from build123d import *

# Parameters (mm, degrees)
SKETCH003_R      = 2
EXTRUDE003_DEPTH = 1.5
SKETCH004_R      = 4
EXTRUDE004_DEPTH = 1.5
EXTRUDE001_DEPTH = 3
SKETCH002_W      = 30
SKETCH002_H      = 30
SKETCH002_R      = 7.071068
EXTRUDE002_DEPTH = 3
SKETCH_W         = 30
SKETCH_H         = 30
EXTRUDE_DEPTH    = 3


with BuildPart() as furo:
    # Sketch003 → Extrude003 (new body)
    with BuildSketch(Plane.XY):
        with Locations((15, 21)):
            Circle(SKETCH003_R)
        with Locations((15, 9)):
            Circle(SKETCH003_R)
    extrude(amount=EXTRUDE003_DEPTH)


with BuildPart() as fusion:
    # Sketch004 → Extrude004 (new body)
    with BuildSketch(Plane.XY.offset(1.5)):
        with Locations((15, 21)):
            Circle(SKETCH004_R)
        with Locations((15, 9)):
            Circle(SKETCH004_R)
    extrude(amount=EXTRUDE004_DEPTH)

    # Fusion: union Furo
    add(furo.part)


with BuildPart() as lateral:
    # Sketch001 → Extrude001 (new body)
    with BuildSketch(Plane.XZ):
        Polygon((0, 3), (0, 30), (30, 3), align=None)
    extrude(amount=-EXTRUDE001_DEPTH)


with BuildPart() as lateral_mirrored:
    # mirror: instance of Lateral
    add(lateral.part.mirror(Plane(origin=(30, 15, 0), x_dir=(-1, 0, 0), z_dir=(0, -1, 0))))


with BuildPart() as frontal:
    # Sketch002 → Extrude002 (new body)
    with BuildSketch(Plane.YZ):
        with Locations((15, 15)):
            Rectangle(SKETCH002_W, SKETCH002_H)
        with Locations((15, 15)):
            Circle(SKETCH002_R, mode=Mode.SUBTRACT)
    extrude(amount=-EXTRUDE002_DEPTH)


with BuildPart() as cut:
    # Sketch → Extrude (new body)
    with BuildSketch(Plane.XY):
        with Locations((15, 15)):
            Rectangle(SKETCH_W, SKETCH_H)
    extrude(amount=EXTRUDE_DEPTH)

    # Fusion001: union Lateral (mirrored), Lateral, Frontal
    add(lateral_mirrored.part)
    add(lateral.part)
    add(frontal.part)

    # Cut: cut Fusion
    add(fusion.part, mode=Mode.SUBTRACT)


solid = cut.part
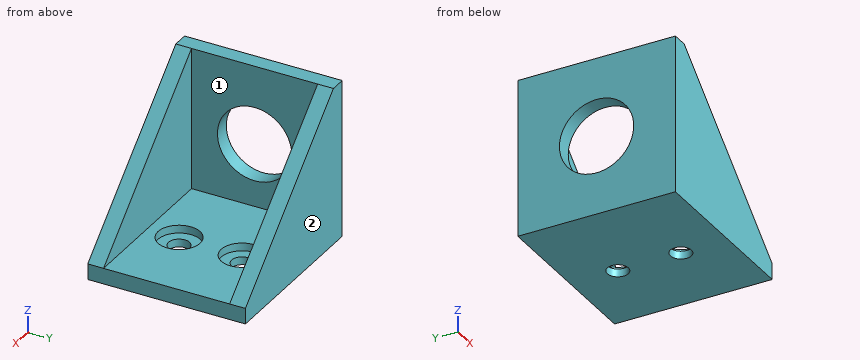
Geometry check sheet. Reference: the model listing, model coordinates, mm. Face numbers are marked on the shaded views. A direction names the side the tool comes from. Coordinates: 2 decimals unless noted, no trailing zeros. Order: outer loops, then holes, each group sorted by start corner. A loop starts at its lowest first (then second) coordinate and runs counter-clockwise, first axis right, second up. Notation, with made-up numbers: (38.25, 25.25) - (85.25, 25.25) arc R19 cw to (85.25, 38.25) - close; hole circle Ø2 at (-4.75, -17.75). An arc over 180 degrees is marked (long way). Answer in a Markdown table with one row per item. Add a question column.
1) Cross-section at B-B, the plane x = 15. Record the cut outline in (y, z), then the cut area to 3 significant figures.
2) Gauge pin test, flat ends, axial feed: P1, Ø3, axis at x = 15, y = 9, coming from the +Z side; P2, Ø8, axis at y = 21.5, z = 21, coming from the +X side; P3, Ø5, axis at x = 18, y = 20.5, coming from the +Z side; P4, Ø6.5, axis at x = 15, y = 21, coming from the +Z side. Record the tip position at first contact, or that the pin passes through.
3) Material ranges on line 1 along Y through (x, z) = (15, 1); line 2 along Y through (x, z) = (15, 2.65); line 3 along Z through (x, y) = (-1.55, 15), recorded low to high. Write a range as [from, to].
4) Cross-section at C-C, the plane z = 21.5. Record the cut outline in (x, y).
5) Set-up check for the marked faces 1 and 2: record each of +Z, -Z, +X, -X, +Y, -Y from which the full face is reachable in a straight line by a thin tool's end or side.
6) Cross-section at D-D, the plane y = 21. Record the cut outline in (x, z), then the cut area to 3 significant figures.
7) Cross-section at A-A, the plane y = 15. Record the cut outline in (x, z).
Check result:
| question | item | result |
|---|---|---|
| 1 | outline | (0, 0) - (7, 0) - (7, 1.5) - (5, 1.5) - (5, 3) - (3, 3) - (3, 16.5) - (0, 16.5) - close; (11, 0) - (19, 0) - (19, 1.5) - (17, 1.5) - (17, 3) - (13, 3) - (13, 1.5) - (11, 1.5) - close; (23, 0) - (30, 0) - (30, 16.5) - (27, 16.5) - (27, 3) - (25, 3) - (25, 1.5) - (23, 1.5) - close |
| 1 | area | 135 mm² |
| 2 | P1 | passes through |
| 2 | P2 | stops at x = 0 |
| 2 | P3 | stops at z = 3 |
| 2 | P4 | stops at z = 1.5 |
| 3 | line 1 | y = [0, 7], [11, 19], [23, 30] |
| 3 | line 2 | y = [0, 5], [13, 17], [25, 30] |
| 3 | line 3 | z = [0, 7.93], [22.07, 30] |
| 4 | outline | (-3, 0) - (9.44, 0) - (9.44, 3) - (0, 3) - (0, 12.22) - (-3, 12.22) - close; (-3, 17.78) - (0, 17.78) - (0, 27) - (9.44, 27) - (9.44, 30) - (-3, 30) - close |
| 5 | face 1 | +Z, +X |
| 5 | face 2 | +Z, -Z, +X, -X, +Y |
| 6 | outline | (-3, 0) - (13, 0) - (13, 1.5) - (11, 1.5) - (11, 3) - (0, 3) - (0, 11.26) - (-3, 11.26) - close; (-3, 18.74) - (0, 18.74) - (0, 30) - (-3, 30) - close; (17, 0) - (30, 0) - (30, 3) - (19, 3) - (19, 1.5) - (17, 1.5) - close |
| 6 | area | 140 mm² |
| 7 | outline | (-3, 0) - (30, 0) - (30, 3) - (0, 3) - (0, 7.93) - (-3, 7.93) - close; (-3, 22.07) - (0, 22.07) - (0, 30) - (-3, 30) - close |
